Geometry check sheet. Reference: the model listing, model coordinates, mm. Give positions to 0.01 mm unless a question says otherwise; leave off trailing zeros. Loops run counter-clockwise (first coordinate to the right, second up) from the corner with the lowest first, then second, coordinate; pieces in that order, holes last.
Autodesk Inventor part; units mm, degrees
ref_plane "YZ Plane" through (0, 0, 0) normal (1, 0, 0) x (0, 1, 0)
ref_plane "XZ Plane" through (0, 0, 0) normal (0, 1, 0) x (-1, 0, 0)
ref_plane "XY Plane" through (0, 0, 0) normal (0, 0, 1) x (1, 0, 0)
sketch "Sketch1" plane through (0, 0, 0) normal (0, 1, 0) x (-1, 0, 0)
  line L0 (4, 4) -> (-4, 4)
  line L1 (-4, 4) -> (-4, -4)
  line L2 (-4, -4) -> (4, -4)
  line L3 (4, -4) -> (4, 4)
  line L4 (4, 4) -> (-4, -4) construction
  line L5 (-4, 4) -> (4, -4) construction
  point P0 (0, 0)
  dimension "d0" = 8
  dimension "d1" = 8
extrude "Extrusion1" add sketch "Sketch1" along normal mid plane 10
fillet "Fillet1" radius 2.5 4 edges at (4, 0, 4) (4, 0, -4) (-4, 0, 4) (-4, 0, -4)
properties part number "Rounded Square"
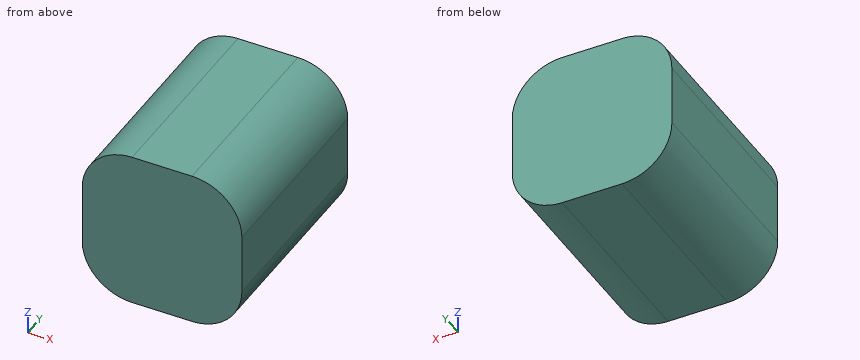
1) Scan lines: line 1 along Z through (x, y) = (-2.5, -2.75); line 2 along X through (y, z) = (4.75, 3.25); line 3 along X through (y, z) = (-0.5, 3). Record each from-to range of solid material in increasing order.
2) Depth check by flat-ended pin: P1, Ø3, axis at x = 3, y = 1, coming from the -Z side; P2, Ø1.5, axis at x = -3, y = 2, coming from the -Z side. Enter the tip coordinate at first touch or a pass-through.
3) Sectioned sample at C-C on z = 3.25. Enter the section's corners in (x, y).
4) Sectioned sample at B-B on x = 3.5. Enter the section's corners in (y, z).
5) Sectioned sample at A-A on y = 4.5. Enter the section's corners in (x, z), plus the area to 3 significant figures.
Determined:
1. line 1: z = -3.79 to 3.79
1. line 2: x = -3.29 to 3.29
1. line 3: x = -3.5 to 3.5
2. P1: stops at z = -4
2. P2: stops at z = -3.88
3. outline: (-3.29, -5) - (3.29, -5) - (3.29, 5) - (-3.29, 5) - close
4. outline: (-5, -3) - (5, -3) - (5, 3) - (-5, 3) - close
5. outline: (-4, -1.5) arc R2.5 ccw to (-1.5, -4) - (1.5, -4) arc R2.5 ccw to (4, -1.5) - (4, 1.5) arc R2.5 ccw to (1.5, 4) - (-1.5, 4) arc R2.5 ccw to (-4, 1.5) - close
5. area: 58.6 mm2
